Geometry check sheet. Reference: drawing and pictorial views, mm from the part's lowest x, y, z. A direction names the side the tool comes from. Give positions to 0.01 mm unless a question says otherwise; leave off trailing zeros. Order: outer loops, then holes, each group sorted by start corner. A loop starts at its lowest first (then second) coordinate and runs counter-clockwise, first axis right, second up. Notation, with made-up numbers: M 31.25,43 L 65.25,43 A15 cw 65.25,55 Z; hole C -16.75,36.25 d6. An arc over 180 degrees is marked long. Answer as CSV lines item,"result". Start each with the question number.
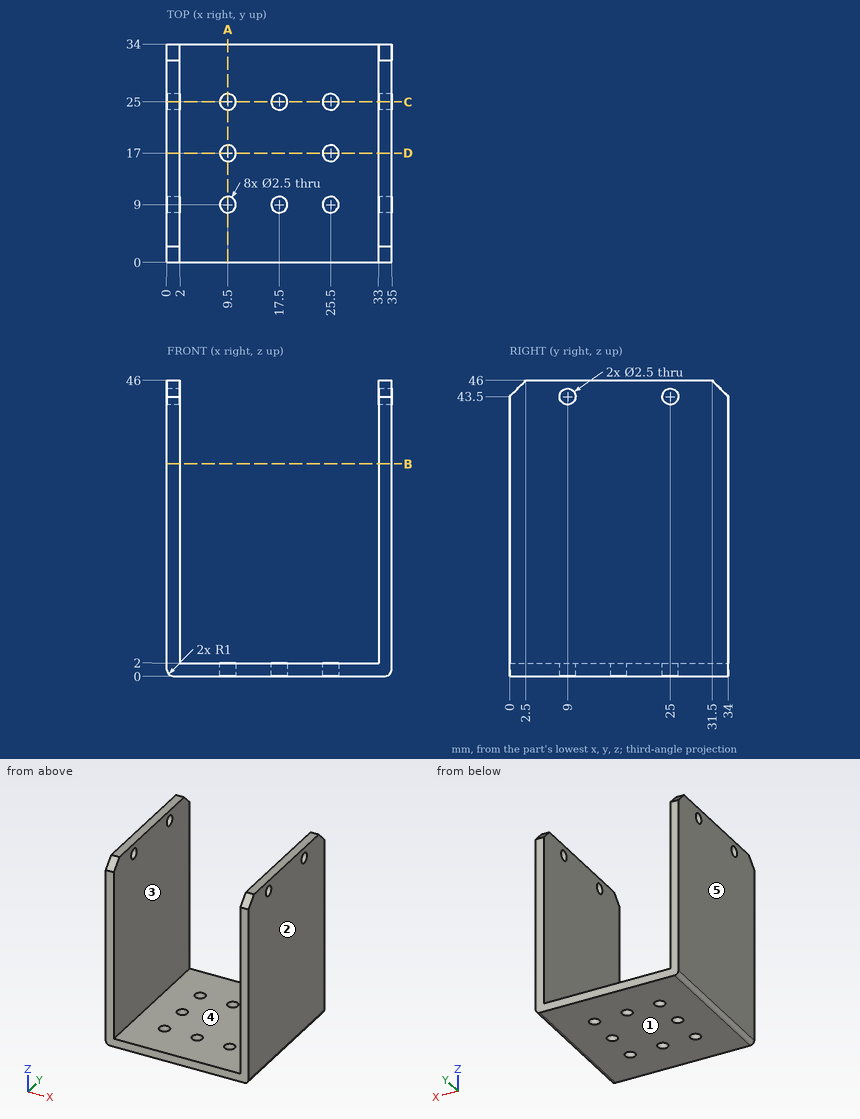
Item 1: Section check B-B on z = 33. Record the boundary of the cut face in (x, y), then the cut area to 3 significant figures.
Item 2: Depth check by flat-ended pin: pin 1 Ø4 at (x, y) = (17.5, 25) entering from +Z. Enter the tip coordinate at first touch or a pass-through.
Item 3: Section check D-D on y = 17. Record the boundary of the cut face in (x, z), then the cut area to 3 significant figures.
Item 4: Scan lines: line 1 along Y through (x, z) = (9.5, 1.25); line 2 along X through (y, z) = (32.5, 22); line 3 along Y through (x, z) = (34, 43.5). Record each from-to range of solid material in increasing order.
Item 5: Draft check along X on the marked faces 1, 2 and 3. Enter one of: pulls with the +X half, pulls with the -X half, needs draft (parallel to the pull), parting line crosses it, or undercut.
Item 6: Section check C-C on y = 25. Give the number of separate pieces and of enclosed holes in the cut face, then the cut area to 3 significant figures.
Item 7: Section check A-A on x = 9.5. Record the boundary of the cut face in (y, z), then the cut area to 3 significant figures.
Item 8: Access from +Z, -Z, +X, -X, +Y, -Y to the whole of each face (thin tool, end or side, straight path). Record for the marked faces 4 and 5.
Numbers:
1,outline,"M 0,0 L 2,0 L 2,34 L 0,34 Z; M 33,0 L 35,0 L 35,34 L 33,34 Z"
1,area,"136 mm2"
2,pin 1,"z = 2"
3,outline,"M 0,1 A1 ccw 1,0 L 8.25,0 L 8.25,2 L 2,2 L 2,46 L 0,46 Z; M 10.75,0 L 24.25,0 L 24.25,2 L 10.75,2 Z; M 26.75,0 L 34,0 A1 ccw 35,1 L 35,46 L 33,46 L 33,2 L 26.75,2 Z"
3,area,"236 mm2"
4,line 1,"0 to 7.75, 10.25 to 15.75, 18.25 to 23.75, 26.25 to 34"
4,line 2,"0 to 2, 33 to 35"
4,line 3,"0 to 7.75, 10.25 to 23.75, 26.25 to 34"
5,face 1,"needs draft"
5,face 2,"pulls with the +X half"
5,face 3,"undercut"
6,separate pieces,"6"
6,enclosed holes,"0"
6,area,"221 mm2"
7,outline,"M 0,0 L 7.75,0 L 7.75,2 L 0,2 Z; M 10.25,0 L 15.75,0 L 15.75,2 L 10.25,2 Z; M 18.25,0 L 23.75,0 L 23.75,2 L 18.25,2 Z; M 26.25,0 L 34,0 L 34,2 L 26.25,2 Z"
7,area,"53.0 mm2"
8,face 4,"+Z, +Y, -Y"
8,face 5,"+Z, -Z, -X, +Y, -Y"
